```python
from build123d import *

# Parameters (mm, degrees)
SKETCH2_W               = 27
SKETCH2_H               = 32
SKETCH2_R               = 9
BOSS_EXTRUDE1_DEPTH     = 6
SKETCH3_W               = 27
SKETCH3_H               = 32
SKETCH3_W_2             = 25
SKETCH3_H_2             = 30
BOSS_EXTRUDE2_DEPTH     = 3
CUT_EXTRUDE1_DEPTH      = 22.77728174
CUT_EXTRUDE1_DEPTH_BACK = 22.77728174
SKETCH1_R               = 1.7
BOSS_EXTRUDE4_REACH     = 24.787
MIRROR2_COPY_1_REACH    = 24.787
SKETCH6_R               = 2.85
CUT_EXTRUDE2_DEPTH      = 4
MIRROR4_COPY_1_SKETCH_R = 2.85
MIRROR4_COPY_1_DEPTH    = 4
FILLET1_R               = 1
FILLET4_R               = 1


with BuildPart() as part:
    # Sketch2 → Boss-Extrude1 (new body)
    with BuildSketch(Plane(origin=(0, 0, 0), x_dir=(1, 0, 0), z_dir=(0, 1, 0))):
        Rectangle(SKETCH2_W, SKETCH2_H)
        with Locations(Location((0, 0, 0), (0, 0, 270))):
            Circle(SKETCH2_R, mode=Mode.SUBTRACT)
    extrude(amount=BOSS_EXTRUDE1_DEPTH)

    # Sketch3 → Boss-Extrude2 (add)
    with BuildSketch(Plane.XZ):
        Rectangle(SKETCH3_W, SKETCH3_H)
        Rectangle(SKETCH3_W_2, SKETCH3_H_2, mode=Mode.SUBTRACT)
    extrude(amount=BOSS_EXTRUDE2_DEPTH)

    # Sketch1 → Cut-Extrude1 (cut, two sides: drawn at the far end of the back side and taken through both)
    with BuildSketch(Plane(origin=(0, 0, 0), x_dir=(1, 0, 0), z_dir=(0, 1, 0)).offset(-CUT_EXTRUDE1_DEPTH_BACK)):
        with Locations((-12.5, 12)):
            Circle(SKETCH1_R)
        with Locations((12.5, 12)):
            Circle(SKETCH1_R)
        with Locations((-12.5, -12)):
            Circle(SKETCH1_R)
        with Locations((12.5, -12)):
            Circle(SKETCH1_R)
    extrude(amount=CUT_EXTRUDE1_DEPTH + CUT_EXTRUDE1_DEPTH_BACK, mode=Mode.SUBTRACT)

    # Sketch5 → Boss-Extrude4 (add, up to next)
    with BuildSketch(Plane.XZ.offset(3), mode=Mode.PRIVATE) as boss_extrude4_sk1:
        with BuildLine():
            Line((13.5, -10.625227292), (13.5, -9.708712153))
            ThreePointArc((13.5, -9.708712153), (10, -12), (13.5, -14.291287847))
            Line((13.5, -14.291287847), (13.5, -13.374772708))
            ThreePointArc((13.5, -13.374772708), (10.8, -12), (13.5, -10.625227292))
        make_face()
    boss_extrude4_tool1 = extrude(boss_extrude4_sk1.sketch, amount=-BOSS_EXTRUDE4_REACH, mode=Mode.PRIVATE) - part.part
    boss_extrude4 = boss_extrude4_tool1.solids().sort_by_distance((13.438967, -3, -10.16697))[0]
    add(boss_extrude4)

    # Mirror1: Boss-Extrude4 across plane
    add(boss_extrude4.mirror(Plane(origin=(0, 0, 0), x_dir=(0, 0, 1), z_dir=(1, 0, 0))))

    # Mirror2: Boss-Extrude4 across plane
    add(boss_extrude4.mirror(Plane.XY))

    # Mirror2 copy 1 sketch → Mirror2 copy 1 (add, up to next)
    with BuildSketch(Plane(origin=(0, -3, 0), x_dir=(-1, 0, 0), z_dir=(0, -1, 0)), mode=Mode.PRIVATE) as mirror2_copy_1_sk1:
        with BuildLine():
            Line((13.5, -10.625227292), (13.5, -9.708712153))
            ThreePointArc((13.5, -9.708712153), (10, -12), (13.5, -14.291287847))
            Line((13.5, -14.291287847), (13.5, -13.374772708))
            ThreePointArc((13.5, -13.374772708), (10.8, -12), (13.5, -10.625227292))
        make_face()
    mirror2_copy_1_tool1 = extrude(mirror2_copy_1_sk1.sketch, amount=-MIRROR2_COPY_1_REACH, mode=Mode.PRIVATE) - part.part
    add(mirror2_copy_1_tool1.solids().sort_by_distance((-13.438967, -3, 10.16697))[0])

    # Sketch6 → Cut-Extrude2 (cut)
    with BuildSketch(Plane(origin=(0, 6, 0), x_dir=(1, 0, 0), z_dir=(0, 1, 0))):
        with Locations((12.5, 12)):
            Circle(SKETCH6_R)
    cut_extrude2 = extrude(amount=-CUT_EXTRUDE2_DEPTH, mode=Mode.SUBTRACT)

    # Mirror3: Cut-Extrude2 across plane
    add(cut_extrude2.mirror(Plane(origin=(0, 0, 0), x_dir=(0, 0, 1), z_dir=(1, 0, 0))), mode=Mode.SUBTRACT)

    # Mirror4: Cut-Extrude2 across plane
    add(cut_extrude2.mirror(Plane.XY), mode=Mode.SUBTRACT)

    # Mirror4 copy 1 sketch → Mirror4 copy 1 (cut)
    with BuildSketch(Plane(origin=(0, 6, 0), x_dir=(-1, 0, 0), z_dir=(0, 1, 0))):
        with Locations((12.5, 12)):
            Circle(MIRROR4_COPY_1_SKETCH_R)
    extrude(amount=-MIRROR4_COPY_1_DEPTH, mode=Mode.SUBTRACT)

    # Fillet1
    fillet1_edges = [part.edges().sort_by_distance(p)[0] for p in [
        (-13.5, 6, -15.334400615),
        (13.5, 6, -15.334400615),
        (0, 6, 16),
        (-13.5, 6, 0),
        (13.5, 6, 0),
        (-13.5, 6, 15.334400615),
        (13.5, 6, 15.334400615),
        (0, 6, -16),
    ]]
    fillet(fillet1_edges, radius=FILLET1_R)

    # Fillet4
    # the kernel refuses this fillet: 1 mm, written as the material it takes off along each edge
    with BuildSketch(Plane(origin=(-12.5, 5, -15), x_dir=(0, 0, -1), z_dir=(-1, 0, 0))) as fillet4_piece_1_section:
        Polygon((0, 0), (FILLET4_R, 0), (FILLET4_R, -FILLET4_R), (0, -FILLET4_R), align=None)
    fillet4_piece_1 = extrude(amount=FILLET4_R, mode=Mode.PRIVATE)
    fillet4_piece_1 = fillet4_piece_1 - Plane(origin=(-12.5, 5, -15), x_dir=(0, -0.7071067811865475, 0.7071067811865475), z_dir=(-1, 0, 0)) * Sphere(FILLET4_R, mode=Mode.PRIVATE)
    add(fillet4_piece_1, mode=Mode.SUBTRACT)
    with BuildSketch(Plane(origin=(12.5, 5, -15), x_dir=(1, 0, 0), z_dir=(0, 0, -1))) as fillet4_piece_2_section:
        Polygon((0, 0), (FILLET4_R, 0), (FILLET4_R, -FILLET4_R), (0, -FILLET4_R), align=None)
    fillet4_piece_2 = extrude(amount=FILLET4_R, mode=Mode.PRIVATE)
    fillet4_piece_2 = fillet4_piece_2 - Plane(origin=(12.5, 5, -15), x_dir=(-0.7071067811865475, -0.7071067811865475, 0), z_dir=(0, 0, -1)) * Sphere(FILLET4_R, mode=Mode.PRIVATE)
    add(fillet4_piece_2, mode=Mode.SUBTRACT)
    with BuildSketch(Plane(origin=(-12.5, 5, 15), x_dir=(-1, 0, 0), z_dir=(0, 0, 1))) as fillet4_piece_3_section:
        Polygon((0, 0), (FILLET4_R, 0), (FILLET4_R, -FILLET4_R), (0, -FILLET4_R), align=None)
    fillet4_piece_3 = extrude(amount=FILLET4_R, mode=Mode.PRIVATE)
    fillet4_piece_3 = fillet4_piece_3 - Plane(origin=(-12.5, 5, 15), x_dir=(0.7071067811865475, -0.7071067811865475, 0), z_dir=(0, 0, 1)) * Sphere(FILLET4_R, mode=Mode.PRIVATE)
    add(fillet4_piece_3, mode=Mode.SUBTRACT)
    with BuildSketch(Plane(origin=(12.5, 5, 15), x_dir=(1, 0, 0), z_dir=(0, 0, 1))) as fillet4_piece_4_section:
        Polygon((0, 0), (FILLET4_R, 0), (FILLET4_R, FILLET4_R), (0, FILLET4_R), align=None)
    fillet4_piece_4 = extrude(amount=FILLET4_R, mode=Mode.PRIVATE)
    fillet4_piece_4 = fillet4_piece_4 - Plane(origin=(12.5, 5, 15), x_dir=(-0.7071067811865475, -0.7071067811865475, 0), z_dir=(0, 0, 1)) * Sphere(FILLET4_R, mode=Mode.PRIVATE)
    add(fillet4_piece_4, mode=Mode.SUBTRACT)
    with BuildSketch(Plane(origin=(13.5, -5.5, -16), x_dir=(-1, 0, 0), z_dir=(0, 1, 0))) as fillet4_piece_5:
        with BuildLine():
            CenterArc((FILLET4_R, FILLET4_R), FILLET4_R, 180, 90)
            Line((0, FILLET4_R), (0, 0))
            Line((0, 0), (FILLET4_R, 0))
        make_face()
    extrude(amount=10.5, mode=Mode.SUBTRACT)
    with BuildSketch(Plane(origin=(13.5, -5.5, 16), x_dir=(-1, 0, 0), z_dir=(0, 1, 0)), Plane(origin=(-13.5, 5, 16), x_dir=(1, 0, 0), z_dir=(0, -1, 0)), Plane(origin=(-13.5, 5, -16), x_dir=(0, 0, 1), z_dir=(0, -1, 0))) as fillet4_piece_6:
        with BuildLine():
            CenterArc((FILLET4_R, -FILLET4_R), FILLET4_R, 90, 90)
            Line((0, -FILLET4_R), (0, 0))
            Line((0, 0), (FILLET4_R, 0))
        make_face()
    extrude(amount=10.5, mode=Mode.SUBTRACT)


solid = part.part
```
For this review, take the finished solid that the model builds, in its own axes (mm). A direction names the side the tool comes from. Round coordinates to 2 decimals unless told otherwise and drop trailing zeros. Write each loop counter-clockwise with the first axis right and the second up, starting at its lowest first coordinate (ties: lowest second). Pieces come first, ordered by that corner, then holes.
1) Take a section at A-A on x = 0. Give the boundary of the cut face in (y, z), then the cut area to 3 significant figures.
Answer below:
outline: (-3, -16) - (5, -16) arc R1 ccw to (6, -15) - (6, -9) - (0, -9) - (0, -15) - (-3, -15) - close; (-3, 15) - (0, 15) - (0, 9) - (6, 9) - (6, 15) arc R1 ccw to (5, 16) - (-3, 16) - close
area: 89.6 mm2
2) Take a section at C-C on z = -4. Give the boundary of the cut face in (x, y), then the cut area to 3 significant figures.
Answer below:
outline: (-13.5, -3) - (-12.5, -3) - (-12.5, 0) - (-8.06, 0) - (-8.06, 6) - (-12.5, 6) arc R1 ccw to (-13.5, 5) - close; (8.06, 0) - (12.5, 0) - (12.5, -3) - (13.5, -3) - (13.5, 5) arc R1 ccw to (12.5, 6) - (8.06, 6) - close
area: 70.8 mm2
3) Insertion check: pin 1 Ø1.9 at (x, z) = (11.5, -12) entering from +Y; pin 2 Ø12.5 at (x, z) = (-6, -2) entering from -Y. Each pin has a flat end and moves straight along its axis. Give the tip position at first contact, or say it passes through.
Answer below:
pin 1: stops at y = 2
pin 2: stops at y = 0
4) Machinability: for faces 5 (the face through (12.5, -1, 0)), 6 (the face through (9.65, 4.03, -12.08)), 7 (the face through (13.5, 0, -14)), which of the approach directions +Z, -Z, +X, -X, +Y, -Y give a long, thin tool a straight path to every point of the face, cutting with its end or side? Answer none if there is none.
Answer below:
face 5: -Y
face 6: +Y
face 7: +Z, -Z, +X, +Y, -Y
5) Take a section at D-D on z = -12. Give the boundary of the cut face in (x, y), then the cut area to 3 significant figures.
Answer below:
outline: (-10.8, -3) - (-10, -3) - (-10, 0) - (10, 0) - (10, -3) - (10.8, -3) - (10.8, 2) - (9.65, 2) - (9.65, 6) - (-9.65, 6) - (-9.65, 2) - (-10.8, 2) - close
area: 125 mm2
6) Take a section at B-B on y = -0.75. Give the boundary of the cut face in (x, z).
Answer below:
outline: (-13.5, -15) arc R1 ccw to (-12.5, -16) - (12.5, -16) arc R1 ccw to (13.5, -15) - (13.5, -13.37) arc R1.7 cw (long way) to (13.5, -10.63) - (13.5, 10.63) arc R1.7 cw (long way) to (13.5, 13.37) - (13.5, 15) arc R1 ccw to (12.5, 16) - (-12.5, 16) arc R1 ccw to (-13.5, 15) - (-13.5, 13.37) arc R1.7 cw (long way) to (-13.5, 10.63) - (-13.5, -10.63) arc R1.7 cw (long way) to (-13.5, -13.37) - close; hole (-12.5, -15) - (12.5, -15) - (12.5, -14.5) arc R2.5 cw to (12.5, -9.5) - (12.5, 9.5) arc R2.5 cw to (12.5, 14.5) - (12.5, 15) - (-12.5, 15) - (-12.5, 14.5) arc R2.5 cw to (-12.5, 9.5) - (-12.5, -9.5) arc R2.5 cw to (-12.5, -14.5) - close
7) Mouldability with a two-part tool opening along X and no side actions: class faces 1 (the face through (-12.5, -1, 0)), 2 (the face through (0, 1, 16)), 3 (the face through (-13.199, 1.056, 15.715)), 4 (the face through (13.5, 1, 0)) as +X half, -X half, draft (parallel to the pull), parting line (faces both ways), or undercut.
Answer below:
face 1: undercut
face 2: draft
face 3: -X half
face 4: +X half
8) For line 1 along Z through (x, y) = (-12.5, 4.9); line 2 along Z through (x, y) = (-12.5, 0.05); line 3 along X through (y, z) = (-0.25, -1.5), list the stretches that pass through material, from the lowest coordinate up.
Answer below:
line 1: z = -16 to -14.85, -9.15 to 9.15, 14.85 to 16
line 2: z = -16 to -13.7, -10.3 to 10.3, 13.7 to 16
line 3: x = -13.5 to -12.5, 12.5 to 13.5
